For this review, take the finished solid that the model builds, in its own axes (mm). A direction names the side the tool comes from. Coordinates: 2 decimals unless noted, no trailing zeros. Write each loop counter-clockwise with the first axis right and the second up, starting at its lowest first coordinate (ties: lowest second). Pieces come first, ordered by that corner, then holes. Notation, with made-up numbers: (-8, -27.75) -> (21, -27.75) arc R30 cw to (21, 8.25) -> close; hole circle Ø9 at (27.25, 72). An arc over 180 degrees is marked (long way). One line per item, written item: value. Start each with the question number.
1) Add section B-B (y = 17). State the section outline as (x, z) points.
2) Machinability: for faces 1 (the flat face through (26.6, -18.9, 5)), 2 (the flat face through (34.05, 24.63, 5.01)), 3 (the flat face through (-20, 7.696, 5)), which of the approach directions +Z, -Z, +X, -X, +Y, -Y give a long, thin tool a straight path to every point of the face, cutting with its end or side? Answer none if there is none.
3) Mouldability with a two-part tool opening along Y and no side actions: class faces 4 (the flat face through (19.364, -22.625, 5.009)), 5 (the cylindrical face through (-41.24, -5.59, 5.15)), 6 (the flat face through (15.103, 24.668, 5.009)) as released by +Y, released by -Y, zero draft, split by the parting line, or undercut.
4) Add section A-A (x = 38). State the section outline as (y, z) points, and give its area (3 significant figures).
5) For pin 1 Ø6 at (y, z) = (9.5, 5.5) entering from -X; pin 2 Ø2 at (y, z) = (-18, 5) entering from +X; pin 3 Ø3 at (x, z) = (46.5, 6) entering from -Y; pin 4 Ø10 at (x, y) = (41.5, -19) entering from +Z, all flat-tipped, find the tip position at first contact; note any pin that passes through.
6) Add section D-D (x = -1). State the section outline as (y, z) points.
7) Add section C-C (z = 3.5). State how many separate pieces and enclosed holes the cut face has, and give its area (3 significant figures).
8) For probe 1 along Y at (x, z) = (-31.5, 3.75); probe 2 along Y at (x, z) = (-5.5, 6); probe 3 along Y at (x, z) = (21, 5.75), list the stretches that pass through material, from the lowest coordinate up. Write a range as from..to.
from build123d import *

# Parameters (mm, degrees)
F0_R        = 6.8863244876
F1_DEPTH    = 10.16
F2_T1_DEPTH = 66.6590982347
F2_T3_DEPTH = 42.201240443
F3_T1_DEPTH = 10.16
F3_T3_DEPTH = 58.4926144872
F3_T5_DEPTH = 51.6908183144
F4_R        = 5.08


# Not quite as in the source:
# - a fillet or chamfer that OpenCascade refuses, or shapes differently, is made with other operations: its cross-section is extruded or revolved along the edge and cut away or added


with BuildPart() as f1:
    # F0 (on Top) → F1 (new body)
    with BuildSketch(Plane.XY):
        Polygon((10.6026988985, 15.246915631), (5.517931655, 10.8906533569), (-3.485009307, 7.6960618608), (-42.6913611591, 7.6960618608), (-42.6913611591, -7.1152271703), (-3.485009307, -7.1152271703), (5.517931655, -10.6002362445), (12.4879479408, -18.1510895491), (19.5621072062, -38.0873594287), (25.8471500129, -38.0873594287), (33.8609059311, -35.2437690269), (36.3021790981, -28.315698728), (32.69538281, -18.1510895491), (36.3021790981, -10.6002362445), (40.0547920587, -9.2686640946), (53.1463883817, -9.2686640946), (59.2151660388, -7.1152271703), (59.2151660388, 5.3727226332), (54.5984730124, 7.6960618608), (40.0547920587, 7.6960618608), (36.3021790981, 10.8906533569), (32.69538281, 15.246915631), (34.4987809541, 27.7348645031), (32.69538281, 32.8171690926), (25.8471500129, 36.0883464863), (19.4785206028, 33.8285105681), align=None)
        Polygon((15.6825426966, -14.9564975873), (22.9429770261, -11.4714885131), (30.3544697336, -26.5248827454), (22.9429770261, -30.0823998534), align=None, mode=Mode.SUBTRACT)
        Polygon((-32.5267501175, -2.7589655947), (-32.5267501175, 4.501469899), (-3.485009307, 4.2110527866), (-3.485009307, -2.7589655947), align=None, mode=Mode.SUBTRACT)
        with Locations((12.1975308284, 0)):
            Circle(F0_R, mode=Mode.SUBTRACT)
        Polygon((51.4038838446, -3.339800518), (26.7184022814, -2.7589655947), (26.7184022814, 3.9206352085), (51.4038838446, 3.9206352085), align=None, mode=Mode.SUBTRACT)
        Polygon((22.9429770261, 7.6960618608), (15.3921246529, 11.7619056255), (22.962263142, 28.9465700275), (29.2712664114, 26.8636122346), align=None, mode=Mode.SUBTRACT)
    extrude(amount=F1_DEPTH)

    # F2: fillet of radius 18.1225687259 on 2 edges, made by hand

    # F2_s2 → F2_t1 (cut)
    with BuildSketch(Plane.XY.offset(-28.2495491174)):
        with BuildLine():
            ThreePointArc((15.7833367489, -27.4380957037), (19.6910161344, -33.825149661), (25.8471500129, -38.0873594287))
            Line((25.8471500129, -38.0873594287), (19.5621072062, -38.0873594287))
            Line((19.5621072062, -38.0873594287), (15.7833367489, -27.4380957037))
        make_face()
    extrude(amount=F2_T1_DEPTH, mode=Mode.SUBTRACT)

    # F2_s4 → F2_t3 (cut)
    with BuildSketch(Plane.XY.offset(-16.0206202215)):
        with BuildLine():
            ThreePointArc((34.1724327506, -34.3596894675), (35.202544115, -28.3169031391), (34.15919812, -22.2763878325))
            Line((34.15919812, -22.2763878325), (36.3021790981, -28.315698728))
            Line((36.3021790981, -28.315698728), (34.1724327506, -34.3596894675))
        make_face()
    extrude(amount=F2_T3_DEPTH, mode=Mode.SUBTRACT)

    # F3: fillet of radius 14.545063472 on 6 edges, made by hand

    # F3_s2 → F3_t1 (join)
    with BuildSketch(Plane.XY):
        with BuildLine():
            ThreePointArc((33.6130817468, 21.6016839559), (33.901548417, 15.9810300876), (36.3021790981, 10.8906533569))
            Line((36.3021790981, 10.8906533569), (32.69538281, 15.246915631))
            Line((32.69538281, 15.246915631), (33.6130817468, 21.6016839559))
        make_face()
        with BuildLine():
            ThreePointArc((36.3021790981, 10.8906533569), (40.5775055267, 8.5179295182), (45.3975437049, 7.6960618608))
            Line((45.3975437049, 7.6960618608), (40.0547920587, 7.6960618608))
            Line((40.0547920587, 7.6960618608), (36.3021790981, 10.8906533569))
        make_face()
        with BuildLine():
            ThreePointArc((35.2695823203, -12.7619848351), (33.8938078195, -17.8922695477), (34.4517445702, -23.1744360815))
            Line((34.4517445702, -23.1744360815), (33.0574978105, -23.5887604555))
            ThreePointArc((33.0574978105, -23.5887604555), (32.7884309604, -22.7627890129), (31.3246156504, -18.6374907295))
            Line((31.3246156504, -18.6374907295), (31.3829198252, -17.5241687984))
            Line((31.3829198252, -17.5241687984), (33.9571193355, -12.1350640844))
            Line((33.9571193355, -12.1350640844), (35.2695823203, -12.7619848351))
        make_face()
        with BuildLine():
            ThreePointArc((40.0547920587, -9.2686640946), (36.4117244984, -12.043489977), (33.8119770372, -15.8134917097))
            Line((33.8119770372, -15.8134917097), (36.3021790981, -10.6002362445))
            Line((36.3021790981, -10.6002362445), (40.0547920587, -9.2686640946))
        make_face()
    extrude(amount=F3_T1_DEPTH)

    # F3_s4 → F3_t3 (cut)
    with BuildSketch(Plane.XY.offset(-24.1663072436)):
        with BuildLine():
            ThreePointArc((59.2151660388, 2.5512957272), (57.6093256229, -4.0921505253), (53.1463883817, -9.2686640946))
            Line((53.1463883817, -9.2686640946), (59.2151660388, -7.1152271703))
            Line((59.2151660388, -7.1152271703), (59.2151660388, 2.5512957272))
        make_face()
    extrude(amount=F3_T3_DEPTH, mode=Mode.SUBTRACT)

    # F3_s6 → F3_t5 (cut)
    with BuildSketch(Plane.XY.offset(-20.7654091572)):
        with BuildLine():
            ThreePointArc((54.5984730124, 7.6960618608), (58.011160428, 2.8609568294), (59.2151660388, -2.9334410297))
            Line((59.2151660388, -2.9334410297), (59.2151660388, 5.3727226332))
            Line((59.2151660388, 5.3727226332), (54.5984730124, 7.6960618608))
        make_face()
    extrude(amount=F3_T5_DEPTH, mode=Mode.SUBTRACT)

    # F4
    f4_edges = [f1.edges().sort_by_distance(p)[0] for p in [
        (-42.691361, 7.696062, 5.08),
        (-42.691361, -7.115227, 5.08),
    ]]
    fillet(f4_edges, radius=F4_R)


solid = f1.part
Numbers:
1. outline: (11.44, 0) -> (17.7, 0) -> (17.7, 10.16) -> (11.44, 10.16) -> close; (26.01, 0) -> (33.68, 0) -> (33.68, 10.16) -> (26.01, 10.16) -> close
2. face 1: +Z, -Z
2. face 2: +Z, -Z, +X
2. face 3: +Z, -Z, -X, +Y
3. face 4: undercut
3. face 5: released by -Y
3. face 6: released by +Y
4. outline: (-10.61, 0) -> (-3.02, 0) -> (-3.02, 10.16) -> (-10.61, 10.16) -> close; (3.92, 0) -> (9.72, 0) -> (9.72, 10.16) -> (3.92, 10.16) -> close
4. area: 136 mm²
5. pin 1: x = -40.89
5. pin 2: x = 33.99
5. pin 3: y = -9.27
5. pin 4: through
6. outline: (-8.08, 0) -> (8.58, 0) -> (8.58, 10.16) -> (-8.08, 10.16) -> close
7. separate pieces: 1
7. enclosed holes: 5
7. area: 1,960 mm²
8. probe 1: -7.12..-2.76, 4.49..7.7
8. probe 2: -7.12..-2.76, 4.23..7.7
8. probe 3: -35.08..-26.03, -12.4..8.74, 24.49..34.37
